```python
from build123d import *

# Parameters (mm, degrees)
SKETCH2_W           = 9
SKETCH2_H           = 11
BOSS_EXTRUDE1_DEPTH = 3.25
BOSS_EXTRUDE2_DEPTH = 10.9
SKETCH4_R           = 3.25
SKETCH4_R_2         = 1
CUT_EXTRUDE1_DEPTH  = 10.9
FILLET1_R           = 0.508


with BuildPart() as part:
    # Sketch2 → Boss-Extrude1 (new body)
    with BuildSketch(Plane.XY):
        Rectangle(SKETCH2_W, SKETCH2_H)
    extrude(amount=BOSS_EXTRUDE1_DEPTH)

    # Sketch3 → Boss-Extrude2 (add)
    with BuildSketch(Plane(origin=(0, 0, 0), x_dir=(-1, 0, 0), z_dir=(0, 0, -1))):
        with BuildLine():
            Line((-4.5, 1), (-3.937, 1))
            ThreePointArc((-3.937, 1), (0, 4.937), (3.937, 1))
            Line((3.937, 1), (4.5, 1))
            Line((4.5, 1), (4.5, -5.5))
            Line((4.5, -5.5), (-4.5, -5.5))
            Line((-4.5, -5.5), (-4.5, 1))
        make_face()
    extrude(amount=BOSS_EXTRUDE2_DEPTH)

    # Sketch4 → Cut-Extrude1 (cut)
    with BuildSketch(Plane.XY.offset(3.25)):
        with Locations((0, 1)):
            Circle(SKETCH4_R)
        with Locations((0, 1)):
            Circle(SKETCH4_R_2, mode=Mode.SUBTRACT)
    extrude(amount=-CUT_EXTRUDE1_DEPTH, mode=Mode.SUBTRACT)

    # Fillet1
    fillet1_edges = [part.edges().sort_by_distance(p)[0] for p in [
        (-1, 1, 3.25),
    ]]
    fillet(fillet1_edges, radius=FILLET1_R)


solid = part.part
```
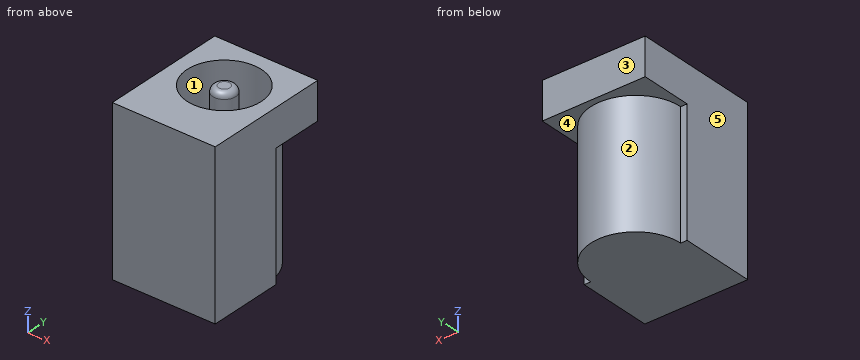
Source: CAD feature listing. Evaluate the final solid. Frame: model axes, mm. Face numbers are marked on the shaded views. A direction names the side the tool comes from. Coordinates: 2 decimals unless noted, no trailing zeros. Loops run counter-clockwise (first coordinate to the right, second up) from the corner with the lowest first, then second, coordinate; pieces in that order, holes last. Notation, with made-up numbers: (12, 45.25) -> (70, 45.25) arc R27 ccw to (70, 84.25) -> close; hole circle Ø6 at (16.25, 33). An arc over 180 degrees is marked (long way). One line per item, written item: value. Start each with the question number.
Q1. Section query C-C, the plane z = 0.5. Return the cut outline in (x, y), and give its area (3 significant figures).
Q2. Section query A-A, the plane z = -7. Return the cut outline in (x, y).
Q3. Line query: line 1 along Y through (x, z) = (0, 0.5); line 2 along Y through (x, z) = (0, -4.75); line 3 along X through (y, z) = (1.75, -2). Output: solid intervals per line, ascending.
Q4. Set-up query: the marked faces 4 and 5. Return all of +Z, -Z, +X, -X, +Y, -Y with unobstructed straight access to the full face (end or side cutting, diameter ignored); none if empty.
Q5. Contact query for flat-ended pins moving along their axis: P1, Ø1.5, axis at x = 1, z = -3.5, coming from the +Y side; P2, Ø0.6, axis at x = -4.5, z = -3.5, coming from the +Y side. Output: stop coordinate, or through.
Q6. Section query D-D, the plane x = 2.25. Return the cut outline in (y, z).
Q7. Mould query, pull axis X, two halves, no side actions, for the marked faces 1, 2 and 3. Classes: pulls with the +X half, pulls with the -X half, needs draft (parallel to the pull), parting line crosses it, or undercut.
Q8. Section query B-B, the plane y = 3.25. Return the cut outline in (x, z), and give its area (3 significant figures).
Results:
1. outline: (-4.5, -5.5) -> (4.5, -5.5) -> (4.5, 5.5) -> (-4.5, 5.5) -> close; circle Ø2 at (0, 1); hole circle Ø6.5 at (0, 1)
1. area: 69.0 mm^2
2. outline: (-4.5, -5.5) -> (4.5, -5.5) -> (4.5, 1) -> (3.94, 1) arc R3.94 ccw to (-3.94, 1) -> (-4.5, 1) -> close; circle Ø2 at (0, 1); hole circle Ø6.5 at (0, 1)
3. line 1: -5.5 to -2.25, 0 to 2, 4.25 to 5.5
3. line 2: -5.5 to -2.25, 0 to 2, 4.25 to 4.94
3. line 3: -3.86 to -3.16, -0.66 to 0.66, 3.16 to 3.86
4. face 4: -Z, +Y
4. face 5: +Z, -Z, -X, +Y, -Y
5. P1: y = 4.93
5. P2: y = 1
6. outline: (-5.5, -10.9) -> (4.23, -10.9) -> (4.23, 0) -> (5.5, 0) -> (5.5, 3.25) -> (3.35, 3.25) -> (3.35, -7.65) -> (-1.35, -7.65) -> (-1.35, 3.25) -> (-5.5, 3.25) -> close
7. face 1: undercut
7. face 2: parting line crosses it
7. face 3: needs draft
8. outline: (-4.5, 0) -> (-3.23, 0) -> (-3.23, -10.9) -> (3.23, -10.9) -> (3.23, 0) -> (4.5, 0) -> (4.5, 3.25) -> (2.35, 3.25) -> (2.35, -7.65) -> (-2.35, -7.65) -> (-2.35, 3.25) -> (-4.5, 3.25) -> close
8. area: 48.6 mm^2
